```python
from build123d import *

# Parameters (mm, degrees)
F0_R     = 5.55
F0_R_2   = 2.55
F1_DEPTH = 10
F2_R     = 5.55
F2_R_2   = 3.6
F3_DEPTH = 10
F4_R     = 1.25
F5_DEPTH = 5.551


with BuildPart() as f1:
    # F0 (on Top) → F1 (new body)
    with BuildSketch(Plane.XY):
        Circle(F0_R)
        Circle(F0_R_2, mode=Mode.SUBTRACT)
    extrude(amount=F1_DEPTH)

    # F2 (on face) → F3 (join)
    with BuildSketch(Plane.XY.offset(10)):
        Circle(F2_R)
        Circle(F2_R_2, mode=Mode.SUBTRACT)
    extrude(amount=F3_DEPTH)

    # F4 (on Right) → F5 (cut, through all)
    with BuildSketch(Plane.YZ):
        with Locations((0, 15)):
            Circle(F4_R)
        with Locations((0, 5)):
            Circle(F4_R)
    extrude(amount=-F5_DEPTH, mode=Mode.SUBTRACT)


solid = f1.part
```
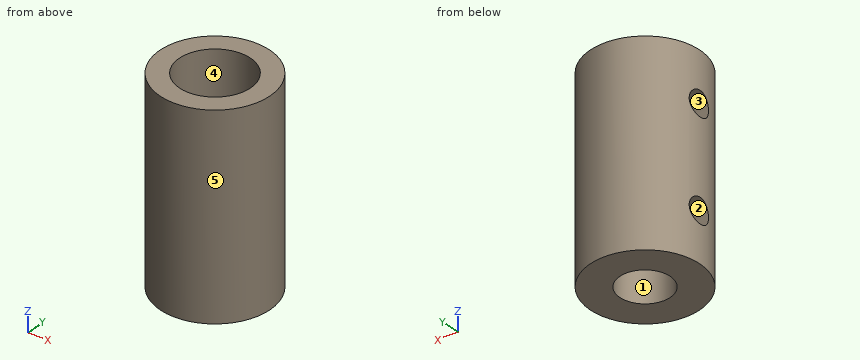
CAD build for the part. Positions are in the model's coordinates, mm. Face numbers are marked on the shaded views. A direction names the side the tool comes from. Coordinates: 2 decimals unless noted, no trailing zeros. Order: outer loops, then holes, each group sorted by start corner. A loop starts at its lowest first (then second) coordinate and runs counter-clockwise, first axis right, second up. Notation, with made-up numbers: (16, -1) -> (33, -1) arc R19 cw to (33, 20) -> close; hole circle Ø7 at (85.5, 26.5). An arc over 180 degrees is marked (long way). Use one line per item in the form item = value. Start each with the question number.
1) Drop flat-ended pins along their axis: pin 1 (2 mm diameter, centred on y = 1.5, z = 6.5, fed in from -X); pin 2 (4.5 mm diameter, centred on x = 0, y = 0, fed in from -Z); pin 3 (4 mm diameter, centred on y = -4, z = 11.5, fed in from -X); pin 4 (3.5 mm diameter, centred on x = 0.5, y = -1.5, fed in from +Z). Give the stop position or say it passes through.
2) Band-saw the part on A-A on y = 0. Give the cut face in (x, z).
3) Tool access for the marked faces 1 and 2: list every direction of +Z, -Z, +X, -X, +Y, -Y with a clear straight run to the whole face (end or side of a thin tool).
4) Pull direction X, two halves, no side cores. Call the marked faces 3, 4 and 5: +X half, -X half, draft (parallel to the pull), parting line (faces both ways), or undercut.
5) Drill centre lines: L1, parallel to X at y = 0, z = 12.75; L2, parallel to X at y = 0, z = 7; L3, parallel to Z at x = 3.25, y = 0.75. Where is each one in solid material? Low to high. Write a range as [from, to].
6) Band-saw the part on D-D on y = -1.75. Give the cut face in (x, z).
7) Band-saw the part on C-C on z = 9.25. Give the cut face in (x, y).
8) Band-saw the part on B-B on x = 0. Give the cut face in (y, z).
Entries:
q1.pin_1 = -5.53
q1.pin_2 = through
q1.pin_3 = -5.18
q1.pin_4 = 10
q2.outline = (-5.55, 0) -> (-2.55, 0) -> (-2.55, 3.75) -> (-5.55, 3.75) -> close; (-5.55, 6.25) -> (-2.55, 6.25) -> (-2.55, 10) -> (-3.6, 10) -> (-3.6, 13.75) -> (-5.55, 13.75) -> close; (-5.55, 16.25) -> (-3.6, 16.25) -> (-3.6, 20) -> (-5.55, 20) -> close; (2.55, 0) -> (5.55, 0) -> (5.55, 20) -> (3.6, 20) -> (3.6, 10) -> (2.55, 10) -> close
q3.face_1 = +Z, -Z
q3.face_2 = -X
q4.face_3 = draft
q4.face_4 = undercut
q4.face_5 = parting line
q5.L1 = [-5.55, -3.6], [3.6, 5.55]
q5.L2 = [-5.55, -2.55], [2.55, 5.55]
q5.L3 = [0, 10]
q6.outline = (-5.27, 0) -> (-1.85, 0) -> (-1.85, 10) -> (-3.15, 10) -> (-3.15, 20) -> (-5.27, 20) -> close; (1.85, 0) -> (5.27, 0) -> (5.27, 20) -> (3.15, 20) -> (3.15, 10) -> (1.85, 10) -> close
q7.outline = circle Ø11.1 at (0, 0); hole circle Ø5.1 at (0, 0)
q8.outline = (-5.55, 0) -> (-2.55, 0) -> (-2.55, 10) -> (-3.6, 10) -> (-3.6, 20) -> (-5.55, 20) -> close; (2.55, 0) -> (5.55, 0) -> (5.55, 20) -> (3.6, 20) -> (3.6, 10) -> (2.55, 10) -> close
